```python
from build123d import *

# Parameters (mm, degrees)
PAD005_DEPTH         = 25
SKETCH010_R          = 1.7
POCKET005_DEPTH      = 7.001
POCKET005_DEPTH_BACK = 9.001
POCKET006_DEPTH      = 3
SKETCH_R             = 1.6
SKETCH_R_2           = 6
PAD_DEPTH            = 4
SKETCH001_R          = 5
PAD001_DEPTH         = 12
SKETCH002_R          = 2.2
POCKET_DEPTH         = 13.001
SKETCH004_R          = 1.5
POCKET002_DEPTH      = 13.001
SKETCH005_R          = 1.5
POCKET003_DEPTH      = 4.001
POCKET003_DEPTH_BACK = 12.001
SKETCH007_R          = 3
SKETCH007_R_2        = 1.5
PAD003_DEPTH         = 2
SKETCH003_R          = 4.75
PAD004_DEPTH         = 2
SKETCH008_R          = 6.25
POCKET004_DEPTH      = 12.001
FILLET_R             = 1.5
FILLET001_R          = 3
FILLET002_R          = 1
FILLET003_R          = 1.49
FILLET004_R          = 3


with BuildPart() as tubeclampingbody:
    # Sketch009 → Pad005 (new body)
    with BuildSketch(Plane.XZ):
        with BuildLine():
            Line((10, 7), (10, -9))
            Line((10, -9), (-10, -9))
            Line((-10, -9), (-10, 7))
            Line((-2, 7), (-10, 7))
            Line((-2, 0), (-2, 7))
            ThreePointArc((-2, 0), (0, -2), (2, 0))
            Line((2, 0), (2, 7))
            Line((2, 7), (10, 7))
        make_face()
    extrude(amount=-PAD005_DEPTH)

    # Sketch010 → Pocket005 (cut, two sides)
    with BuildSketch(Plane.XY) as pocket005_sk:
        with Locations((-5, 5)):
            Circle(SKETCH010_R)
        with Locations((5, 5)):
            Circle(SKETCH010_R)
        with Locations((-5, 20)):
            Circle(SKETCH010_R)
        with Locations((5, 20)):
            Circle(SKETCH010_R)
    extrude(amount=POCKET005_DEPTH, mode=Mode.SUBTRACT)
    extrude(pocket005_sk.sketch, amount=-POCKET005_DEPTH_BACK, mode=Mode.SUBTRACT)

    # Sketch011 (on DatumPlane) → Pocket006 (cut)
    with BuildSketch(Plane.XY.offset(-9)):
        Polygon((-2.125, 3.340118), (-2.125, 6.659882), (-5, 8.319764), (-7.875, 6.659882), (-7.875, 3.340118), (-5, 1.680236), align=None)
        Polygon((7.875, 3.340118), (7.875, 6.659882), (5, 8.319764), (2.125, 6.659882), (2.125, 3.340118), (5, 1.680236), align=None)
        Polygon((-2.125, 18.340118), (-2.125, 21.659882), (-5, 23.319764), (-7.875, 21.659882), (-7.875, 18.340118), (-5, 16.680236), align=None)
        Polygon((7.875, 18.340118), (7.875, 21.659882), (5, 23.319764), (2.125, 21.659882), (2.125, 18.340118), (5, 16.680236), align=None)
    extrude(amount=POCKET006_DEPTH, mode=Mode.SUBTRACT)


with BuildPart() as tubeclampingbody_1:
    # Body001 placement: moved
    add(tubeclampingbody.part.moved(Location((5.5, 20, 5))))


with BuildPart() as drivebase_refined:
    # Sketch → Pad (new body)
    with BuildSketch(Plane.XY):
        Polygon((0, 20), (-26, 20), (-26, 0), (-26, -20), (0, -20), (20, -20), (20, 0), (20, 20), align=None)
        with Locations((-23, 5.9)):
            Circle(SKETCH_R, mode=Mode.SUBTRACT)
        with Locations((-23, -5.9)):
            Circle(SKETCH_R, mode=Mode.SUBTRACT)
        Circle(SKETCH_R_2, mode=Mode.SUBTRACT)
    extrude(amount=-PAD_DEPTH)

    # Sketch001 → Pad001 (join)
    with BuildSketch(Plane.XY):
        with Locations((13, -13)):
            Circle(SKETCH001_R)
        Polygon((0, 20), (20, 20), (20, 7), (0, 7), (-20, 7), (-20, 20), align=None)
    extrude(amount=PAD001_DEPTH)

    # Sketch002 (on DatumPlane) → Pocket (cut, through all)
    with BuildSketch(Plane.XZ.offset(-7)):
        with Locations((5.5, 5)):
            Circle(SKETCH002_R)
    extrude(amount=-POCKET_DEPTH, mode=Mode.SUBTRACT)

    # Sketch004 (on DatumPlane) → Pocket002 (cut, through all)
    with BuildSketch(Plane.XZ.offset(-7)):
        with Locations((-12, 5)):
            Circle(SKETCH004_R)
    extrude(amount=-POCKET002_DEPTH, mode=Mode.SUBTRACT)

    # Sketch005 → Pocket003 (cut, two sides)
    with BuildSketch(Plane.XY) as pocket003_sk:
        with Locations((13, -13)):
            Circle(SKETCH005_R)
        with Locations((13, 13)):
            Circle(SKETCH005_R)
    extrude(amount=-POCKET003_DEPTH, mode=Mode.SUBTRACT)
    extrude(pocket003_sk.sketch, amount=POCKET003_DEPTH_BACK, mode=Mode.SUBTRACT)

    # Sketch007 (on DatumPlane) → Pad003 (join)
    with BuildSketch(Plane.XZ.offset(-7)):
        with Locations((5.5, 5)):
            Circle(SKETCH007_R)
        with Locations((5.5, 5)):
            Circle(SKETCH007_R_2, mode=Mode.SUBTRACT)
    extrude(amount=PAD003_DEPTH)

    # Sketch003 (on DatumPlane) → Pad004 (join)
    with BuildSketch(Plane.XZ.offset(-7)):
        with BuildLine():
            ThreePointArc((-7.465411, 0), (-12, 11.75), (-16.534589, 0))
            Line((-16.534589, 0), (-7.465411, 0))
        make_face()
        with Locations((-12, 5)):
            Circle(SKETCH003_R, mode=Mode.SUBTRACT)
    extrude(amount=PAD004_DEPTH)

    # Sketch008 → Pocket004 (cut, through all)
    with BuildSketch(Plane.XY):
        Circle(SKETCH008_R)
    extrude(amount=POCKET004_DEPTH, mode=Mode.SUBTRACT)

    # Fillet
    fillet_edges = [drivebase_refined.edges().sort_by_distance(p)[0] for p in [
        (8, -13, 0),
    ]]
    fillet(fillet_edges, radius=FILLET_R)

    # Fillet001
    fillet001_edges = [drivebase_refined.edges().sort_by_distance(p)[0] for p in [
        (-26, -20, -2),
        (20, -20, -2),
        (20, 20, -2),
        (-26, 20, -2),
        (20, 7, 6),
        (-20, 20, 6),
    ]]
    fillet(fillet001_edges, radius=FILLET001_R)

    # Fillet002
    fillet002_edges = [drivebase_refined.edges().sort_by_distance(p)[0] for p in [
        (-20, 7, 6),
    ]]
    fillet(fillet002_edges, radius=FILLET002_R)

    # Fusion: union TubeClampingBody
    add(tubeclampingbody_1.part)

    # Fillet003
    fillet003_edges = [drivebase_refined.edges().sort_by_distance(p)[0] for p in [
        (-4.5, 20, 6),
        (15.5, 20, 6),
    ]]
    fillet(fillet003_edges, radius=FILLET003_R)

    # Fillet004
    fillet004_edges = [drivebase_refined.edges().sort_by_distance(p)[0] for p in [
        (-4.5, 45, 4),
        (15.5, 45, 4),
    ]]
    fillet(fillet004_edges, radius=FILLET004_R)


solid = drivebase_refined.part
```
CAD build for the part. Positions are in the model's coordinates, mm. A direction names the side the tool comes from. Coordinates: 2 decimals unless noted, no trailing zeros. Order: outer loops, then holes, each group sorted by start corner. A loop starts at its lowest first (then second) coordinate and runs counter-clockwise, first axis right, second up. Notation, with made-up numbers: M 18,-3 L 66,-3 A27 ccw 66,22 Z; hole C 2.5,54 d6. An arc over 180 degrees is marked long. Answer as CSV lines item,"result".
1) Cut at C-C (y = 0). List the corners of the cut face in (x, z), then the cut area to 3 significant figures.
Verdict:
outline,"M -26,-4 L -6,-4 L -6,0 L -26,0 Z; M 6,-4 L 20,-4 L 20,0 L 6,0 Z"
area,"136 mm2"
2) Mould opens along Y. For faces 1 (the flat face through (3.375, 25, -3)), 2 (the cylindrical face through (4.3, 6, 4.1)), 3 (the flat face through (-12, 20, 2)) say: released by +Y, released by -Y, zero draft, split by the parting line, or undercut.
Verdict:
face 1,"undercut"
face 2,"zero draft"
face 3,"released by +Y"
3) Cut at D-D (y = 18). List the corners of the cut face in (x, z).
Verdict:
outline,"M -25.83,-4 L 19.83,-4 L 19.83,12 L -19.83,12 L -19.83,0 L -25.83,0 Z; hole C -12,5 d3; hole C 5.5,5 d4.4"
4) Drill centre lines: L1, parallel to Y at x = 0.5, z = 7.5; L2, parallel to Y at x = -23, z = -2.8; L3, parallel to X at y = 40, z = 7.25. Where is each one in solid material? Low to high. Write a range as from..to.
Verdict:
L1,"7..23.3, 26.7..38.3, 41.7..45"
L2,"-20..-7.5, -4.3..4.3, 7.5..20"
L3,"-4.5..-1.2, 2.2..3.5, 7.5..8.8, 12.2..15.5"
5) Cut at A-A (y = -13). List the corners of the cut face in (x, z).
Verdict:
outline,"M -26,-4 L 11.5,-4 L 11.5,12 L 8,12 L 8,1.5 A1.5 cw 6.5,0 L -26,0 Z; M 14.5,-4 L 20,-4 L 20,0 L 19.5,0 A1.5 cw 18,1.5 L 18,12 L 14.5,12 Z"
6) Cut at B-B (x = -12). List the corners of the cut face in (y, z).
Verdict:
outline,"M -20,-4 L 20,-4 L 20,3.5 L 7,3.5 L 7,0.25 L 5,0.25 L 5,0 L -20,0 Z; M 5,9.75 L 7,9.75 L 7,6.5 L 20,6.5 L 20,12 L 7,12 L 7,11.75 L 5,11.75 Z"
7) 3-axis set-ups, long thin cutter, end or side, ignore diameter. For faces 4 (the flat face through (7.5, 32, 8)), 5 (the flat face through (7, 7, 6)), 6 (the flat face through (9.08, 42.5, -2.52)): which of +Z, -Z, +X, -X, +Y, -Y reach the whole face in a straight line?
Verdict:
face 4,"+Z, +Y"
face 5,"none"
face 6,"-Z"
8) Flat gauge pins, fed straight in: P1, Ø0.9, axis at y = 24, z = -2, coming from the -X side; P2, Ø1.7, axis at x = 1.5, y = 41, coming from the -Z side; P3, Ø5, axis at x = -12, z = 5, coming from the +Y side. Where does each tip first touch, or does it go through?
Verdict:
P1,"x = -4.5"
P2,"z = -1"
P3,"y = 20"
